from build123d import *

# Parameters (mm, degrees)
SKETCH1_W                        = 44.45
SKETCH1_H                        = 44.45
SKETCH1_W_2                      = 38.1
SKETCH1_H_2                      = 38.1
BOSS_EXTRUDE1_DEPTH              = 914.4
F_17_64_0_26563_DIAMETER_HOLE1_D = 6.747002


with BuildPart() as part:
    # Sketch1 → Boss-Extrude1 (new body)
    with BuildSketch(Plane.XY):
        Rectangle(SKETCH1_W, SKETCH1_H)
        Rectangle(SKETCH1_W_2, SKETCH1_H_2, mode=Mode.SUBTRACT)
    extrude(amount=BOSS_EXTRUDE1_DEPTH)

    # 17/64 (0.26563) Diameter Hole1 (through all)
    with Locations(Plane(origin=(0, 22.225, 0), x_dir=(1, 0, 0), z_dir=(0, 1, 0))):
        with Locations((0, -38.1), (0, -876.3), (0, -317.5), (0, -596.9), (0, -114.3), (0, -342.9), (0, -571.5), (0, -800.1)):
            Hole(F_17_64_0_26563_DIAMETER_HOLE1_D / 2)


solid = part.part
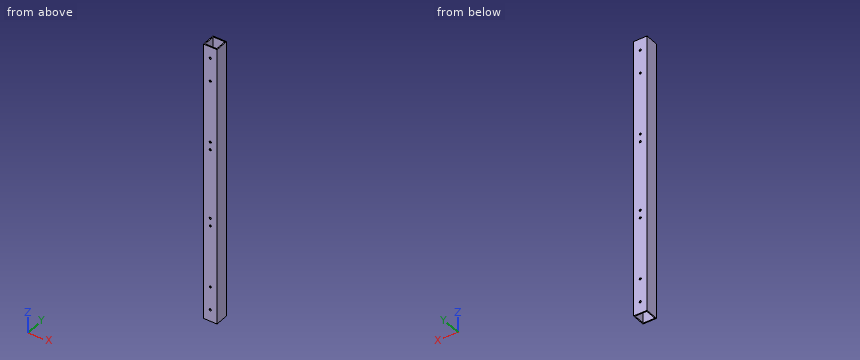
The model under review builds one solid part; all positions refer to its coordinate system, in mm. Give positions to 0.01 mm unless a question says otherwise; leave off trailing zeros. Write each loop counter-clockwise with the first axis right and the second up, starting at its lowest first coordinate (ties: lowest second). Pieces come first, ordered by that corner, then holes. Notation, with made-up numbers: M -14,61.25 L -1,61.25 A31 ccw -1,91.25 Z; hole C -35,-22.5 d9. An arc over 180 degrees is marked long. One line per question, with ' | ' between items. Start each with the question number.
Item 1: We need section C-C on z = 680. Write out the cut boundary in (x, y) (3 decimals).
Item 2: For pin 1 (8 mm diameter, centred on x = 0, z = 38.1, fed in from -Y) (3 decimals); pin 2 (6 mm diameter, centred on x = 0, z = 571.5, fed in from +Y), all flat-tipped, find the tip position at first contact; note any pin that passes through.
Item 3: Wall thickness on line 1 (X direction, y = 15, z = 222) (3 decimals); line 2 (X direction, y = 20, z = 342) (3 decimals): over which ranges is each line inside the solid? List them lowest first. Write a range as from..to.
Item 4: We need section A-A on x = -11. Write out the cut boundary in (y, z) (3 decimals).
Results found:
1) outline: M -22.225,-22.225 L 22.225,-22.225 L 22.225,22.225 L -22.225,22.225 Z; hole M -19.05,-19.05 L 19.05,-19.05 L 19.05,19.05 L -19.05,19.05 Z
2) pin 1: stops at y = -22.225 | pin 2: passes through
3) line 1: x = -22.225..-19.05, 19.05..22.225 | line 2: x = -22.225..-3.251, 3.251..22.225
4) outline: M -22.225,0 L -19.05,0 L -19.05,914.4 L -22.225,914.4 Z; M 19.05,0 L 22.225,0 L 22.225,914.4 L 19.05,914.4 Z
